The listing builds one solid part. Answer for the finished solid, in the listing's coordinates (mm). Face numbers are marked on the shaded views. A direction names the side the tool comes from. Round coordinates to 2 decimals unless told otherwise and drop trailing zeros. Order: outer loops, then holes, each group sorted by start corner. A loop starts at its lowest first (then second) coordinate and runs counter-clockwise, first axis right, second up. Notation, with made-up numbers: (73, 6.5) - (122, 6.5) arc R24 cw to (122, 45.5) - close; hole circle Ø3 at (-13, -22.75). An arc over 180 degrees is marked (long way). Write item = value, one per line.
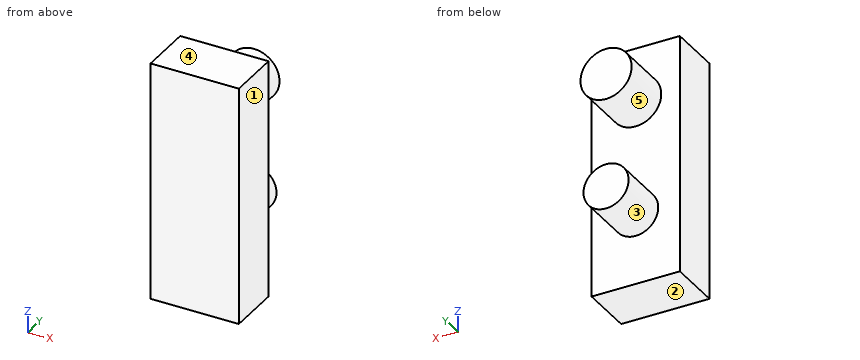
Autodesk Inventor part; units mm, degrees
ref_plane "YZ Plane" through (0, 0, 0) normal (1, 0, 0) x (0, 1, 0)
ref_plane "XZ Plane" through (0, 0, 0) normal (0, 1, 0) x (-1, 0, 0)
ref_plane "XY Plane" through (0, 0, 0) normal (0, 0, 1) x (1, 0, 0)
sketch "Sketch1" plane through (0, 0, 0) normal (0, 1, 0) x (-1, 0, 0)
  line L0 (0, 0) -> (8.2727, 0)
  line L1 (8.2727, 0) -> (8.2727, -22.4672)
  line L2 (8.2727, -22.4672) -> (0, -22.4672)
  line L3 (0, -22.4672) -> (0, 0)
  circle A0 centre (4.1364, -5.0346) radius 2.3953
  circle A1 centre (4.1364, -15.7692) radius 2.113
extrude "Extrusion1" add sketch "Sketch1" along normal blind 5
extrude "Extrusion2" add sketch "Sketch1" along normal blind 10 contours A0 | A1
properties part number ","
Q1. Section B-B on x = -1.5 is taken. Determine the outline of the cut face in (y, z).
Model answer:
outline = (0, -22.47) - (5, -22.47) - (5, 0) - (0, 0) - close
Q2. Find the intervals of material crossed by line 1 (Y direction, x = -7, z = -14.25); line 2 (Z direction, x = -2.5, y = 8.5); line 3 (Z direction, x = -3.5, y = 5.5), in increasing order. Write a range as from..to.
Model answer:
line_1 = 0..5
line_2 = -17.11..-14.43, -6.78..-3.29
line_3 = -17.78..-13.75, -7.34..-2.73
Q3. Section C-C on y = 9.5 is taken. Determine the outline of the cut face in (x, z), then the cut area to 3 significant figures.
Model answer:
outline = circle Ø4.79 at (-4.14, -5.03); circle Ø4.23 at (-4.14, -15.77)
area = 32.1 mm^2
Q4. Flat-ended cylindrical pins translate along their axes: P1, Ø2, axis at x = -3, y = 9, coming from the -Z side; P2, Ø2, axis at y = 8.5, z = -5.5, coming from the +X side; P3, Ø3, axis at x = -4, z = -11.5, coming from the +Y side. Find the tip coordinate at first contact, or state that the pin passes through.
Model answer:
P1 = -17.88
P2 = -1.74
P3 = 5
Q5. Section D-D on z = -4 is taken. Determine the outline of the cut face in (x, y).
Model answer:
outline = (-8.27, 0) - (0, 0) - (0, 5) - (-1.98, 5) - (-1.98, 10) - (-6.3, 10) - (-6.3, 5) - (-8.27, 5) - close
Q6. Section A-A on z = -7 is taken. Determine the outline of the cut face in (x, y).
Model answer:
outline = (-8.27, 0) - (0, 0) - (0, 5) - (-2.77, 5) - (-2.77, 10) - (-5.51, 10) - (-5.51, 5) - (-8.27, 5) - close
Q7. For the marked faces 4 and 5, determine the directions among +Z, -Z, +X, -X, +Y, -Y from which every point of the face is accessible in a straight line to the end or side of a thin tool.
Model answer:
face_4 = +Z, +X, -X, +Y, -Y
face_5 = +Y
Q8. Determine the mould class of the marked faces 1, 2 and 3 for opening direction Z: released by +Z, released by -Z, zero draft, split by the parting line, or undercut.
Model answer:
face_1 = zero draft
face_2 = released by -Z
face_3 = undercut
